Source: CAD feature listing. Evaluate the final solid. Frame: model axes, mm. A direction names the side the tool comes from. Give positions to 0.01 mm unless a question says otherwise; leave off trailing zeros. Order: outer loops, then holes, each group sorted by start corner. A loop starts at its lowest first (then second) coordinate and runs counter-clockwise, first axis right, second up.
1) Draft query along Y for faces 1 (the face through (-2, -15, 1)), 2 (the face through (59, -35, 2)), 3 (the face through (-2, -5, 1)), 4 (the face through (0, -3, 1)). Return one class per face: released by +Y, released by -Y, zero draft, split by the parting line, or undercut.
2) Section B-B, the plane y = -22. Return loops of the section in (x, z).
3) Section A-A, the plane z = 2.1. Return loops of the section in (x, y), plus the area to 3 significant figures.
4) Material intervals for line 1 (X direction, y = -19, z = 1.85), sorted ascending.
5) Access query for faces 5 (the face through (122, -5, 2)), 6 (the face through (122, -15, 2)), 7 (the face through (-2, -25, 1)). Directions: +Z, -Z, +X, -X, +Y, -Y. A direction counts if a zero-diameter tool reaches every point of the face in a straight line with its end or side. Return the directions, or none.
6) First-contact query: P1, Ø0.9, axis at x = -1.5, z = 1.5, coming from the +Y side; P2, Ø0.9, axis at y = -20.5, z = 2, coming from the +X side. Flat tips, straight axial feed; report the tip coordinate or a pass-through.
```python
from build123d import *

# Parameters (mm, degrees)
ESQUISSE1_W                = 119.98
ESQUISSE1_H                = 35
BOSS_EXTRU_1_DEPTH         = 3
ESQUISSE2_W                = 3
ESQUISSE2_H                = 10
BOSS_EXTRU_2_DEPTH         = 5
R_P_TITION_LIN_AIRE1_COUNT = 2
R_P_TITION_LIN_AIRE1_PITCH = 20
ESQUISSE3_W                = 3
ESQUISSE3_H                = 10
BOSS_EXTRU_3_DEPTH         = 5
R_P_TITION_LIN_AIRE2_COUNT = 2
R_P_TITION_LIN_AIRE2_PITCH = 20


with BuildPart() as part:
    # Esquisse1 → Boss.-Extru.1 (new body)
    with BuildSketch(Plane.XY):
        with Locations((59.99, -17.5)):
            Rectangle(ESQUISSE1_W, ESQUISSE1_H)
    extrude(amount=BOSS_EXTRU_1_DEPTH)

    # Esquisse2 → Boss.-Extru.2 (add)
    with BuildSketch(Plane.ZY):
        with Locations((1.5, -30)):
            Rectangle(ESQUISSE2_W, ESQUISSE2_H)
    boss_extru_2 = extrude(amount=BOSS_EXTRU_2_DEPTH)

    # Répétition linéaire1: Boss.-Extru.2 ×2
    with Locations(*[(0, i * R_P_TITION_LIN_AIRE1_PITCH, 0) for i in range(1, R_P_TITION_LIN_AIRE1_COUNT)]):
        add(boss_extru_2)

    # Esquisse3 → Boss.-Extru.3 (add)
    with BuildSketch(Plane(origin=(119.98, 0, 0), x_dir=(0, 0, -1), z_dir=(1, 0, 0))):
        with Locations((-1.5, -30)):
            Rectangle(ESQUISSE3_W, ESQUISSE3_H)
    boss_extru_3 = extrude(amount=BOSS_EXTRU_3_DEPTH)

    # Répétition linéaire2: Boss.-Extru.3 ×2
    with Locations(*[(0, i * R_P_TITION_LIN_AIRE2_PITCH, 0) for i in range(1, R_P_TITION_LIN_AIRE2_COUNT)]):
        add(boss_extru_3)


solid = part.part
```
From the geometry:
1. face 1: undercut
1. face 2: released by -Y
1. face 3: released by +Y
1. face 4: zero draft
2. outline: (0, 0) - (119.98, 0) - (119.98, 3) - (0, 3) - close
3. outline: (-5, -35) - (124.98, -35) - (124.98, -25) - (119.98, -25) - (119.98, -15) - (124.98, -15) - (124.98, -5) - (119.98, -5) - (119.98, 0) - (0, 0) - (0, -5) - (-5, -5) - (-5, -15) - (0, -15) - (0, -25) - (-5, -25) - close
3. area: 4,400 mm2
4. line 1: x = 0 to 119.98
5. face 5: +Z, -Z, +X, +Y
5. face 6: +Z, -Z, +X
5. face 7: +Z, -Z, -X
6. P1: stops at y = -5
6. P2: stops at x = 119.98
